from build123d import *

# Parameters (mm, degrees)
SKETCH1_W                = 80
SKETCH1_H                = 40
BOSS_EXTRUDE1_DEPTH      = 5
SKETCH2_W                = 5
SKETCH2_H                = 40
BOSS_EXTRUDE2_DEPTH      = 20
SKETCH3_W                = 5
SKETCH3_H                = 40
BOSS_EXTRUDE3_DEPTH      = 20
SKETCH4_W                = 5
SKETCH4_H                = 10
CUT_EXTRUDE1_DEPTH       = 3
SKETCH5_W                = 5
SKETCH5_H                = 10
CUT_EXTRUDE2_DEPTH       = 3
M3_CLEARANCE_HOLE1_D     = 3.4
M3_CLEARANCE_HOLE1_DEPTH = 5
M3_CLEARANCE_HOLE1_TIP   = 1.021463052


with BuildPart() as part:
    # Sketch1 → Boss-Extrude1 (new body)
    with BuildSketch(Plane(origin=(0, 0, 0), x_dir=(1, 0, 0), z_dir=(0, 1, 0))):
        Rectangle(SKETCH1_W, SKETCH1_H)
    extrude(amount=BOSS_EXTRUDE1_DEPTH)

    # Sketch2 → Boss-Extrude2 (add)
    with BuildSketch(Plane(origin=(0, 5, 0), x_dir=(1, 0, 0), z_dir=(0, 1, 0))):
        with Locations((-37.5, 0)):
            Rectangle(SKETCH2_W, SKETCH2_H)
    extrude(amount=BOSS_EXTRUDE2_DEPTH)

    # Sketch3 → Boss-Extrude3 (add)
    with BuildSketch(Plane(origin=(0, 5, 0), x_dir=(1, 0, 0), z_dir=(0, 1, 0))):
        with Locations((37.5, 0)):
            Rectangle(SKETCH3_W, SKETCH3_H)
    extrude(amount=BOSS_EXTRUDE3_DEPTH)

    # Sketch4 → Cut-Extrude1 (cut)
    with BuildSketch(Plane(origin=(0, 25, 0), x_dir=(1, 0, 0), z_dir=(0, 1, 0))):
        with Locations((-37.5, 15)):
            Rectangle(SKETCH4_W, SKETCH4_H)
        with Locations((-37.5, -15)):
            Rectangle(SKETCH4_W, SKETCH4_H)
    extrude(amount=-CUT_EXTRUDE1_DEPTH, mode=Mode.SUBTRACT)

    # Sketch5 → Cut-Extrude2 (cut)
    with BuildSketch(Plane(origin=(0, 25, 0), x_dir=(1, 0, 0), z_dir=(0, 1, 0))):
        with Locations((37.5, -15)):
            Rectangle(SKETCH5_W, SKETCH5_H)
        with Locations((37.5, 15)):
            Rectangle(SKETCH5_W, SKETCH5_H)
    extrude(amount=-CUT_EXTRUDE2_DEPTH, mode=Mode.SUBTRACT)

    # M3 Clearance Hole1
    with Locations(Plane(origin=(0, 0, 0), x_dir=(-1, 0, 0), z_dir=(0, -1, 0))):
        with Locations((37.5, -17.5), (37.5, 17.5), (-37.5, 17.5), (-37.5, -17.5)):
            Hole(M3_CLEARANCE_HOLE1_D / 2, depth=M3_CLEARANCE_HOLE1_DEPTH)
            with Locations((0, 0, -(M3_CLEARANCE_HOLE1_DEPTH + M3_CLEARANCE_HOLE1_TIP / 2))):  # 118° drill point
                Cone(0, M3_CLEARANCE_HOLE1_D / 2, M3_CLEARANCE_HOLE1_TIP, mode=Mode.SUBTRACT)


solid = part.part
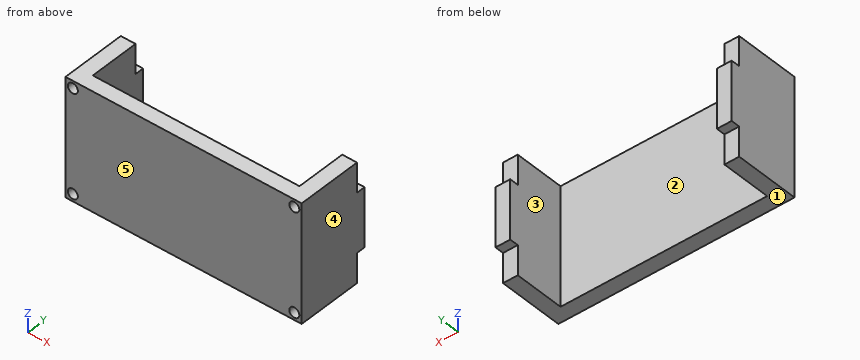
Source: CAD feature listing. Evaluate the final solid. Frame: model axes, mm. Face numbers are marked on the shaded views. A direction names the side the tool comes from. Coordinates: 2 decimals unless noted, no trailing zeros. Loops run counter-clockwise (first coordinate to the right, second up) from the corner with the lowest first, then second, coordinate; pieces in that order, holes last. Notation, with made-up numbers: (13, 82) - (44, 82) arc R36 cw to (44, 118) - close; hole circle Ø1 at (-7.5, 13). An arc over 180 degrees is marked (long way). Return JSON: item names as keys, results as strings.
Q1. Material intervals for line 1 along Z through (x, y) = (-37.5, 2.3); line 2 along X through (y, z) = (3.8, -17.5); line 3 along Z through (x, y) = (36, 1.5), sorted ascending.
Results:
{"line 1": "-20 to -19.2, -15.8 to 15.8, 19.2 to 20", "line 2": "-40 to -39.2, -35.8 to 35.8, 39.2 to 40", "line 3": "-20 to -18.3, -16.7 to 16.7, 18.3 to 20"}
Q2. Section B-B, the plane z = -12. Return loops of the section in (x, y), plus the area to 3 significant figures.
Results:
{"outline": "(-40, 0) - (40, 0) - (40, 22) - (35, 22) - (35, 5) - (-35, 5) - (-35, 22) - (-40, 22) - close", "area": "570 mm2"}
Q3. Contact query for flat-ended pins moving along their axis: P1, Ø3, axis at x = -37.5, z = -17.5, coming from the -Y side; P2, Ø5.5, axis at x = 38.5, z = 13.5, coming from the +Y side; P3, Ø0.9, axis at x = -37.5, y = 23.5, coming from the +Z side. Output: stop coordinate, or through.
Results:
{"P1": "y = 5.12", "P2": "y = 22", "P3": "z = 10"}
Q4. Mould query, pull axis X, two halves, no side actions, for the marked faces 3, 4 and 5. Classes: released by +X, released by -X, zero draft, split by the parting line, or undercut.
Results:
{"face 3": "undercut", "face 4": "released by +X", "face 5": "zero draft"}
Q5. Access query for the marked faces 1 and 2. Directions: +Z, -Z, +X, -X, +Y, -Y. A direction counts if a zero-diameter tool reaches every point of the face in a straight line with its end or side. Return the directions, or none.
Results:
{"face 1": "-Z, +X, -X, +Y, -Y", "face 2": "+Z, -Z, +Y"}
Q6. Section A-A, the plane y = 13.25. Return loops of the section in (x, z).
Results:
{"outline": "(-40, -20) - (-35, -20) - (-35, 20) - (-40, 20) - close; (35, -20) - (40, -20) - (40, 20) - (35, 20) - close"}
Q7. Section C-C, the plane x = 34. Return loops of the section in (y, z), plus the area to 3 significant figures.
Results:
{"outline": "(0, -20) - (5, -20) - (5, 20) - (0, 20) - close", "area": "200 mm2"}
